Geometry check sheet. Reference: the model listing, model coordinates, mm. A direction names the side the tool comes from. Give positions to 0.01 mm unless a question says otherwise; leave off trailing zeros. Write each loop counter-clockwise with the first axis right and the second up, starting at its lowest first coordinate (ties: lowest second). Pieces come first, ordered by that corner, then holes. Notation, with made-up numbers: (-37, 41) - (18, 41) arc R26 ccw to (18, 76) - close; hole circle Ø7 at (49.25, -20.5). An arc over 180 degrees is marked (long way). One line per question, with ' | ' between items. Start each with the question number.
Q1. Gauge pin test, flat ends, axial feed: P1, Ø8, axis at x = -10, z = 21, coming from the -Y side; P2, Ø4, axis at x = 12, z = 2.5, coming from the +Y side; P3, Ø4, axis at x = 11, z = 19.5, coming from the +Y side. Record the tip position at first contact, or that the pin passes through.
Q2. Section check C-C on y = 9.75. Count the separate pieces of the cut face and the enclosed holes in it, and give its area (3 significant figures).
Q3. Section check A-A on x = -10. Record the boundary of the cut face in (y, z) (3 decimals).
Q4. Section check B-B on z = 21. Record the boundary of the cut face in (x, y) (3 decimals).
Q5. Section check D-D on z = 0. Record the boundary of the cut face in (x, y).
Q6. Release check for a two-part mould opening along Z. For faces 1 (the face through (23, 9, 29)), 2 (the face through (-25, 7, 0)), 3 (the face through (-12.28, 12.26, 23.49)) record: +Z half, -Z half, draft (parallel to the pull), parting line (faces both ways), or undercut.
Q7. Thickness scan on L1, parallel to Z at x = -7, y = 1.25 (3 decimals); L2, parallel to X at y = 3.25, z = 22.5 (3 decimals); L3, parallel to Z at x = -10, y = 9. Record the ranges inside material, lowest first. Write a range as [from, to].
Q8. Set-up check for faces 4 (the face through (-3.499, 6.503, 0.253)), 5 (the face through (-4, 7, 30)), 6 (the face through (-10, 3, -26.715)): record each of +Z, -Z, +X, -X, +Y, -Y from which the full face is reachable in a straight line by a thin tool's end or side.
Autodesk Inventor part; units mm, degrees
ref_plane "Work Plane2" through (11, 18, -30) normal (1, 0, 0) x (0, 1, 0)
ref_plane "XZ Plane" through (0, 0, 0) normal (0, 1, 0) x (-1, 0, 0)
ref_plane "XY Plane" through (0, 0, 0) normal (0, 0, 1) x (1, 0, 0)
sketch "Sketch1" plane through (0, 0, 0) normal (0, 1, 0) x (-1, 0, 0)
  line L0 (-25, 30) -> (25, 30)
  line L1 (25, 30) -> (25, -30)
  line L2 (25, -30) -> (-25, -30)
  line L3 (-25, -30) -> (-25, 30)
  line L4 (-25, 30) -> (25, -30) construction
  line L5 (25, 30) -> (-25, -30) construction
  point P0 (0, 0)
  dimension "d0" = 50
  dimension "d1" = 60
extrude "Extrusion1" add sketch "Sketch1" along normal blind 18
sketch "Sketch2" plane through (25, 0, 30) normal (1, 0, 0) x (0, 0, -1)
  line L0 (60, 18) -> (0, 18)
  circle A0 centre (30, 18) radius 9.5
  point P0 (30, 0)
  point P1 (20.5, 18)
  point P2 (39.5, 18)
  dimension "d4" = 19
extrude "Extrusion2" cut sketch "Sketch2" against normal through all contours A0 L0 picked at (28.8771, 15.0391)
sketch "Sketch3" plane through (25, 0, -30) normal (0, 0, -1) x (-1, 0, 0)
  line L0 (0, 18) -> (50, 18)
  circle A0 centre (14, 18) radius 10
  point P0 (25, 0)
  point P1 (24, 18)
  point P2 (4, 18)
  dimension "d7" = 20
  dimension "d8" = 14
extrude "Extrusion3" cut sketch "Sketch3" against normal through all contours L0 A0 picked at (12.1065, 15.2567)
sketch "Sketch4" plane through (0, 0, 0) normal (0, 0, 1) x (1, 0, 0)
  arc A0 (1, 18) -> (21, 18) centre (11, 18) ccw
  circle A1 centre (11, 18) radius 11.5
  point P0 (0, 0)
  dimension "d11" = 23
extrude "Extrusion4" cut sketch "Sketch4" along normal mid plane 39
ref_plane "Work Plane2" through (11, 18, -30) normal (1, 0, 0) x (0, 1, 0)
sketch "Sketch5" plane through (11, 18, -30) normal (1, 0, 0) x (0, 1, 0)
  arc A0 (0, 39.5) -> (0, 20.5) centre (0, 30) ccw
  circle A1 centre (0, 30) radius 11.5
  point P0 (-18, 30)
  dimension "d14" = 23
extrude "Extrusion5" cut sketch "Sketch5" against normal blind 24
sketch "Sketch7" plane through (0, 0, 0) normal (0, -1, 0) x (1, 0, 0)
  line L0 (25, -30) -> (-25, -30)
  line L1 (-25, 30) -> (25, 30)
  line L2 (-25, -30) -> (-25, 30)
  point P0 (0, 0)
  point P1 (-10, -21)
  point P2 (-10, 21)
  dimension "d28" = 9
  dimension "d29" = 9
  dimension "d30" = 15
hole "Hole2" at (-10, 0, -21) at (-10, 0, 21) direction (0, 1, 0) diameter 6.756 end through all
fillet "Fillet1" radius 5 4 edges at (-25, 9, -30) (-25, 9, 30) (25, 9, 30) (25, 9, -30)
sketch "Sketch8" plane through (0, 0, 0) normal (0, -1, 0) x (1, 0, 0)
  circle A0 centre (-10, -21) radius 3.378
  circle A1 centre (-10, 21) radius 3.378
  line L0 (-4.285, -26.715) -> (-15.715, -26.715)
  line L1 (-15.715, -26.715) -> (-15.715, -15.285)
  line L2 (-15.715, -15.285) -> (-4.285, -15.285)
  line L3 (-4.285, -15.285) -> (-4.285, -26.715)
  line L4 (-4.285, -26.715) -> (-15.715, -15.285) construction
  line L5 (-15.715, -26.715) -> (-4.285, -15.285) construction
  line L6 (-4.285, 26.715) -> (-15.715, 26.715)
  line L7 (-15.715, 26.715) -> (-15.715, 15.285)
  line L8 (-15.715, 15.285) -> (-4.285, 15.285)
  line L9 (-4.285, 15.285) -> (-4.285, 26.715)
  line L10 (-4.285, 26.715) -> (-15.715, 15.285) construction
  line L11 (-15.715, 26.715) -> (-4.285, 15.285) construction
  point P0 (0, 0)
  dimension "d39" = 11.43
  dimension "d40" = 11.43
  dimension "d41" = 11.43
  dimension "d42" = 11.43
extrude "Extrusion6" cut sketch "Sketch8" against normal blind 6.35
equation "\"d40\" = d39"
equation "\"d41\" = d39"
equation "\"d42\" = d40"
properties part number "Valve Block Top"
Working result:
1) P1: stops at y = 6.35 | P2: stops at y = 6.9 | P3: stops at y = 8.2
2) separate pieces: 4 | enclosed holes: 2 | area: 1,620 mm2
3) outline: (0, -30) - (18, -30) - (18, -24.378) - (6.35, -24.378) - (6.35, -26.715) - (0, -26.715) - close; (0, -15.285) - (6.35, -15.285) - (6.35, -17.622) - (18, -17.622) - (18, -11.5) arc R11.5 cw to (18, 11.5) - (18, 17.622) - (6.35, 17.622) - (6.35, 15.285) - (0, 15.285) - close; (0, 26.715) - (6.35, 26.715) - (6.35, 24.378) - (18, 24.378) - (18, 30) - (0, 30) - close
4) outline: (-25, 0) - (-15.715, 0) - (-15.715, 6.35) - (-13.378, 6.35) - (-13.378, 18) - (-25, 18) - close; (-6.622, 6.35) - (-4.285, 6.35) - (-4.285, 0) - (25, 0) - (25, 18) - (21, 18) arc R10 cw to (1, 18) - (-6.622, 18) - close
5) outline: (-25, 0) - (25, 0) - (25, 8.5) - (17.48, 8.5) arc R11.5 cw to (11, 6.5) - (-13, 6.5) - (-13, 8.5) - (-25, 8.5) - close
6) face 1: +Z half | face 2: draft | face 3: undercut
7) L1: z = [-30, -26.715], [-15.285, 15.285], [26.715, 30] | L2: x = [-25, -15.715], [-4.285, 25] | L3: z = [-30, -24.38], [-17.62, -7.16], [7.16, 17.62], [24.38, 30]
8) face 4: +Y | face 5: +Z, +X, -X, +Y, -Y | face 6: -Y
